Can you work these out from the model? Positions are in its coordinate system, mm. A direction names the side the tool comes from. Give positions to 0.01 mm unless a question says otherwise; leave off trailing zeros. Order: outer loops, then holes, each group sorted by start corner. A loop starts at its lowest first (then second) coordinate and runs counter-clockwise, first axis right, second up. Notation, with made-up numbers: (81, 35.25) - (136, 35.25) arc R33 cw to (136, 65.25) - close; hole circle Ø1 at (-27.75, -3.75). An arc over 180 degrees is marked (long way). Return JSON: item names as keys, results as strings.
Autodesk Inventor part; units mm, degrees
ref_plane "Work Plane1" through (-28.8888, 50.8, -330.2) normal (1, 0, 0) x (0, 0, -1)
ref_plane "YZ Plane" through (0, 0, 0) normal (1, 0, 0) x (0, 1, 0)
ref_plane "XZ Plane" through (0, 0, 0) normal (0, 1, 0) x (-1, 0, 0)
sketch "Sketch1" plane through (0, 0, 0) normal (0, 1, 0) x (-1, 0, 0)
  line L0 (0, 0) -> (0, -330.2)
  line L1 (0, -330.2) -> (0, -122.0086)
  line L2 (0, -330.2) -> (28.8888, -330.2)
  line L3 (28.8888, -330.2) -> (0, 0)
  dimension "d0" = 330.2
  dimension "d1" = 5
extrude "Extrusion1" add sketch "Sketch1" along normal blind 50.8
ref_plane "Work Plane1" through (-28.8888, 50.8, -330.2) normal (1, 0, 0) x (0, 0, -1)
sketch "Sketch2" plane through (0, 0, 0) normal (1, 0, 0) x (0, 0, -1)
  line L0 (0, 0) -> (330.2, 0)
  line L1 (0, 50.8) -> (330.2, 50.8)
  line L2 (0, 0) -> (330.2, 0)
  line L3 (330.2, 0) -> (330.2, 50.8)
  line L4 (330.2, 50.8) -> (0, 50.8)
  line L5 (0, 50.8) -> (0, 0)
extrude "Extrusion2" add sketch "Sketch2" along normal blind 9.8552
sketch "Sketch4" plane through (-28.8888, 50.8, -330.2) normal (1, 0, 0) x (0, 0, -1)
  line L0 (0, -50.8) -> (0, 0) construction
  line L1 (0, -25.4) -> (-279.4, -25.4) construction
  line L2 (0, -50.8) -> (-330.2, -50.8) construction
  line L3 (-330.2, -50.8) -> (-330.2, 0) construction
  point P0 (-254, -25.4)
  point P1 (-50.8, -25.4)
  point P2 (-330.2, 0)
  dimension "d16" = 25.4
  dimension "d17" = 76.2
  dimension "d18" = 279.4
hole "Hole2" at (-28.8888, 25.4, -76.2) at (-28.8888, 25.4, -279.4) direction (1, 0, 0) diameter 6.7564 end through all counterbore diameter 17.78 counterbore depth 27.94
equation "\"d0\" = lengthOfFixture"
equation "\"d1\" = cutAngle"
equation "\"d2\" = heightOfJig"
equation "\"d4\" = addedDepthToSupportBolts"
equation "\"d16\" = heightOfBoltHolt"
equation "\"lengthOfFixture\" = 330.2"
equation "\"cutAngle\" = 5deg"
equation "\"bottomToFirstHole\" = 76.2"
equation "\"distanceBetweenBolts\" = 203.2"
equation "\"bottomToSecondHole\" = bottomToFirstHole + distanceBetweenBolts"
equation "\"heightOfBoltHolt\" = 25.4"
equation "\"boltSize\" = 6.35"
equation "\"heightOfJig\" = 50.8"
equation "\"addedDepthToSupportBolts\" = 9.8552"
properties part number "jigForRipCuts"
1. Suppose I cut it at C-C (z = -76.2). List the corners of the cut face in (x, y) for me, plus the area to 3 significant figures.
Checks:
{"outline": "(-6.67, 0) - (9.86, 0) - (9.86, 22.02) - (-0.95, 22.02) - (-0.95, 16.51) - (-6.67, 16.51) - close; (-6.67, 34.29) - (-0.95, 34.29) - (-0.95, 28.78) - (9.86, 28.78) - (9.86, 50.8) - (-6.67, 50.8) - close", "area": "665 mm^2"}
2. Suppose I cut it at D-D (y = 43.5). List the corners of the cut face in (x, z) for me.
Checks:
{"outline": "(-28.89, -330.2) - (9.86, -330.2) - (9.86, 0) - (0, 0) - close"}
3. For pin 1 Ø11 at (y, z) = (25.4, -279.4) entering from -X; pin 2 Ø19.5 at (y, z) = (23.5, -278.5) entering from -X; pin 3 Ø19.5 at (y, z) = (25.5, -72.5) entering from -X, each with a flat end and sliding along its axis, tell me the tip position at first contact or that it passes through.
Checks:
{"pin 1": "x = -0.95", "pin 2": "x = -25.22", "pin 3": "x = -6.72"}
4. Suppose I cut it at B-B (y = 25.4). List the corners of the cut face in (x, z) for me.
Checks:
{"outline": "(-28.89, -330.2) - (9.86, -330.2) - (9.86, -282.78) - (-0.95, -282.78) - (-0.95, -288.29) - (-25.22, -288.29) - close; (-23.67, -270.51) - (-0.95, -270.51) - (-0.95, -276.02) - (9.86, -276.02) - (9.86, -79.58) - (-0.95, -79.58) - (-0.95, -85.09) - (-7.44, -85.09) - close; (-5.89, -67.31) - (-0.95, -67.31) - (-0.95, -72.82) - (9.86, -72.82) - (9.86, 0) - (0, 0) - close"}
5. On a 3-axis mill with a long thin cutter (end or side, diameter ignored), from which of +Z, -Z, +X, -X, +Y, -Y can I reach the whole of each face in a straight line? I mean faces 1 (the face through (-12.92, 25.01, -288.28)), 2 (the face through (4.529, 24.385, -276.178)). Say none if no direction works.
Checks:
{"face 1": "-X", "face 2": "+X, -X"}
6. Thinking about a two-plate mould opening in Y: for faces 3 (the face through (-0.949, 25.3, -275.6)), 4 (the face through (-5, 0, -199)), 5 (the face through (9.855, 26, -163)), which applies, +Y half, -Y half, draft (parallel to the pull), parting line (faces both ways), or undercut?
Checks:
{"face 3": "undercut", "face 4": "-Y half", "face 5": "draft"}
7. If I drill on L1, parallel to Z at x = 1, y = 25; L2, parallel to Y at x = -3, z = -76.2; L3, parallel to X at y = 38, z = -69, over which ranges is the centre line in solid material (lowest first)? Write a range as [from, to].
Checks:
{"L1": "[-330.2, -282.75], [-276.05, -79.55], [-72.85, 0]", "L2": "[0, 16.51], [34.29, 50.8]", "L3": "[-6.04, 9.86]"}
8. Suppose I cut it at A-A (z = -279.4). List the corners of the cut face in (x, y) for me, plus the area to 3 significant figures.
Checks:
{"outline": "(-24.44, 0) - (9.86, 0) - (9.86, 22.02) - (-0.95, 22.02) - (-0.95, 16.51) - (-24.44, 16.51) - close; (-24.44, 34.29) - (-0.95, 34.29) - (-0.95, 28.78) - (9.86, 28.78) - (9.86, 50.8) - (-24.44, 50.8) - close", "area": "1,250 mm^2"}
